Print and shaded views of the part. All mm, measured from the part's lowest x, y and z. A direction names the side the tool comes from. Coordinates: 2 decimals unless noted, no trailing zeros. Loops run counter-clockwise (first coordinate to the right, second up) from the corner with the lowest first, then second, coordinate; pieces in that order, holes last.
1) Two-plate mould, pull along X, no slides. Class the marked faces 4, 5 and 6: +X half, -X half, draft (parallel to the pull), parting line (faces both ways), or undercut.
2) Saw through at B-B, the plane x = 2. Write the cut outline in (y, z).
3) Pin check, flat tips, straight feed: pin 1 Ø5 at (x, z) = (6.5, 7) entering from +Y; pin 2 Ø6 at (x, y) = (4.5, 4) entering from +Z; pin 3 Ø8 at (x, z) = (15, 12) entering from +Y; pin 4 Ø1.5 at (x, y) = (19.5, 3.5) entering from -Z. Stop position of each tip, or through.
4) Saw through at A-A, the plane y = 7.5. Write the cut outline in (x, z).
5) Wall check: line 1 along Z through (x, y) = (3, 7.35); line 2 along Z through (x, y) = (9.5, 7.75); line 3 along X through (y, z) = (7, 11.75). Give the ranges that are in metal, low to high.
6) Which spindle directions (+Z, -Z, +X, -X, +Y, -Y) get a long thin tool onto all of the face, cutting with end or side? Do the marked faces 1, 2 and 3. Say none if no direction does.
7) Saw through at C-C, the plane z = 7. Write the cut outline in (x, y).
8) Saw through at D-D, the plane x = 7.5. Write the cut outline in (y, z).
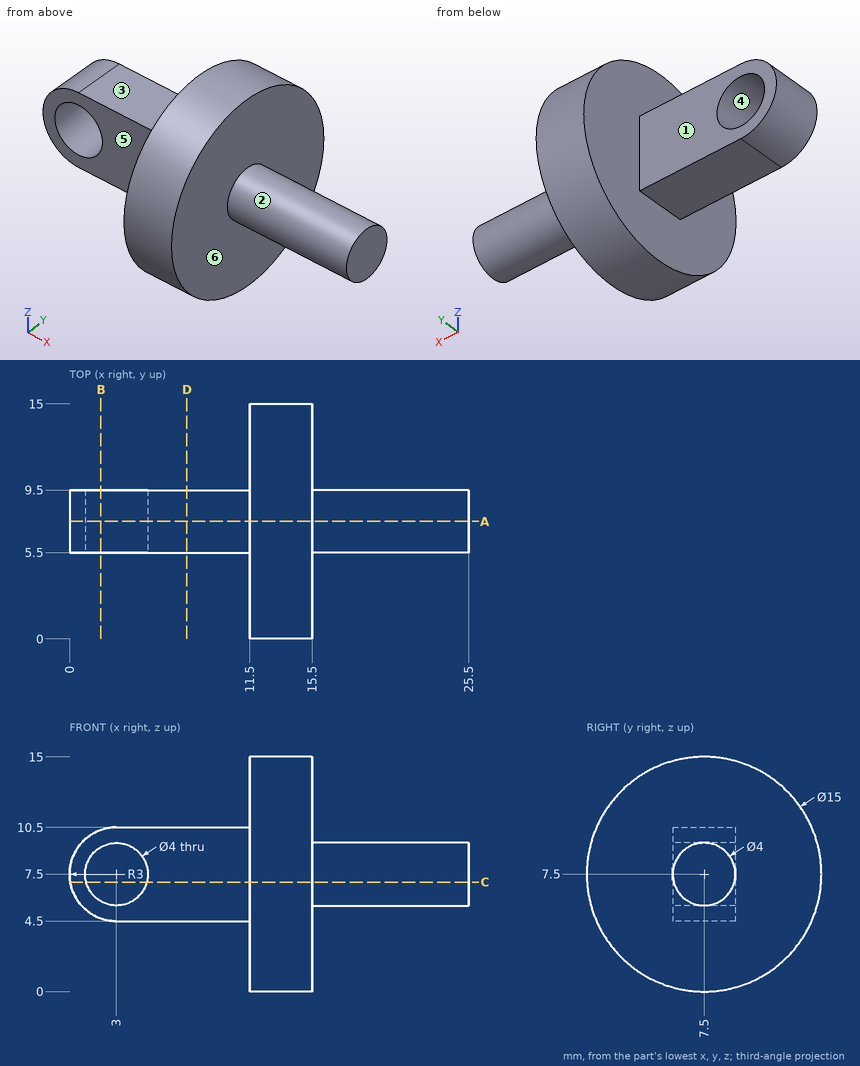
Data:
1. face 4: undercut
1. face 5: draft
1. face 6: +X half
2. outline: (5.5, 4.67) - (9.5, 4.67) - (9.5, 5.77) - (5.5, 5.77) - close; (5.5, 9.23) - (9.5, 9.23) - (9.5, 10.33) - (5.5, 10.33) - close
3. pin 1: stops at y = 9.5
3. pin 2: stops at z = 10.5
3. pin 3: stops at y = 14.98
3. pin 4: passes through
4. outline: (3, 4.5) - (11.5, 4.5) - (11.5, 0) - (15.5, 0) - (15.5, 5.5) - (25.5, 5.5) - (25.5, 9.5) - (15.5, 9.5) - (15.5, 15) - (11.5, 15) - (11.5, 10.5) - (3, 10.5) arc R3 ccw to start; hole circle Ø4 at (3, 7.5)
5. line 1: z = 4.5 to 5.5, 9.5 to 10.5
5. line 2: z = 4.5 to 10.5
5. line 3: x = 11.5 to 15.5
6. face 1: +Z, -Z, -X, +Y
6. face 2: +X
6. face 3: +Z, -X, +Y, -Y
7. outline: (0.04, 5.5) - (1.06, 5.5) - (1.06, 9.5) - (0.04, 9.5) - close; (4.94, 5.5) - (11.5, 5.5) - (11.5, 0.02) - (15.5, 0.02) - (15.5, 5.56) - (25.5, 5.56) - (25.5, 9.44) - (15.5, 9.44) - (15.5, 14.98) - (11.5, 14.98) - (11.5, 9.5) - (4.94, 9.5) - close
8. outline: (5.5, 4.5) - (9.5, 4.5) - (9.5, 10.5) - (5.5, 10.5) - close
